Can you work these out from the model? Positions are in its coordinate system, mm. A direction names the side the tool comes from. Round coordinates to 2 decimals unless told otherwise and drop trailing zeros. Write each loop counter-clockwise with the first axis right and the second up, starting at its lowest first coordinate (ties: lowest second). Pieces come first, ordered by that corner, then holes. Notation, with made-up numbers: M -17.75,33 L 13.25,33 A16 cw 13.25,56 Z; hole C -3.75,27 d1. An arc over 180 degrees is marked long. Answer as a JSON object with one key per item and string values. Group by question number.
1) On a 3-axis mill with a long thin cutter (end or side, diameter ignored), from which of +Z, -Z, +X, -X, +Y, -Y can I reach the whole of each face in a straight line? I mean faces 1 (the cylindrical face through (78.108, 594.894, 0.28)), 2 (the flat face through (380, -469, -17)). Say none if no direction works.
2) Suppose I cut it at A-A, the plane x = 0. Write out the boundary of the cut face in (y, z), and give its area (3 significant figures).
3) I'm going to push flat-ended pins straight in: pin 1 Ø2 at (x, z) = (-210.5, -7.5) entering from +Y; pin 2 Ø6 at (x, z) = (-345.5, 2) entering from -Y; pin 3 Ø5 at (y, z) = (240.5, -9) entering from -X. Where does each tip first touch, or does it pass through?
4) Suppose I cut it at C-C, the plane z = -8.5. Write out the boundary of the cut face in (x, y).
5) Please list where these lines run through material, in increasing order: L1, parallel to Y at x = 0, z = -4; L2, parallel to X at y = -16.5, z = 10; L3, parallel to X at y = -449, z = 10. Write a range as [from, to].
6) If we mould it in two halves opening along Z, with no side actions, what happens to faces 3 (the flat face through (-187, 572, -20)), 4 (the flat face through (-187, 572, 20)), 5 (the flat face through (380, -469, 17)), 6 (the cylindrical face through (138.74, -624.78, 0.28))? For each: +Z half, -Z half, draft (parallel to the pull), parting line (faces both ways), or undercut.
from build123d import *

# Parameters (mm, degrees)
F0_W   = 40
F0_H   = 40
F0_W_2 = 34
F0_H_2 = 34


with BuildPart() as f1:
    # F0 (on Front) → F1 (revolve)
    with BuildSketch(Plane.XZ):
        with Locations((-620, 0)):
            Rectangle(F0_W, F0_H)
        with Locations((-620, 0)):
            Rectangle(F0_W_2, F0_H_2, mode=Mode.SUBTRACT)
    revolve(axis=Axis((0, 0, -37.583534), (0, 0, -1)))


solid = f1.part
Results:
{
 "1": {"face 1": "+Z, -Z", "face 2": "none"},
 "2": {"outline": "M -640,-20 L -600,-20 L -600,20 L -640,20 Z; M 600,-20 L 640,-20 L 640,20 L 600,20 Z; hole M -637,-17 L -603,-17 L -603,17 L -637,17 Z; hole M 603,-17 L 637,-17 L 637,17 L 603,17 Z", "area": "888 mm^2"},
 "3": {"pin 1": "y = 604.74", "pin 2": "y = -540.64", "pin 3": "x = -594.1"},
 "4": {"outline": "C 0,0 d1280; C 0,0 d1206; hole C 0,0 d1274; hole C 0,0 d1200"},
 "5": {"L1": "[-640, -637], [-603, -600], [600, 603], [637, 640]", "L2": "[-639.79, -636.79], [-602.77, -599.77], [599.77, 602.77], [636.79, 639.79]", "L3": "[-456.07, -451.85], [-402.5, -397.99], [397.99, 402.5], [451.85, 456.07]"},
 "6": {"face 3": "-Z half", "face 4": "+Z half", "face 5": "undercut", "face 6": "draft"}
}
